```python
from build123d import *

# Parameters (mm, degrees)
F1_DEPTH = 15


with BuildPart() as f1:
    # F0 (on Top) → F1 (new body)
    with BuildSketch(Plane.XY):
        with BuildLine():
            Line((-28, 8), (-28, 0))
            Line((-28, 0), (22, 0))
            Line((22, 0), (22, 8))
            ThreePointArc((22, 8), (21.414214, 9.414214), (20, 10))
            Line((20, 10), (12, 10))
            ThreePointArc((12, 10), (10.585786, 10.585786), (10, 12))
            Line((10, 12), (10, 31))
            ThreePointArc((10, 31), (6.485281, 39.485281), (-2, 43))
            Line((-2, 43), (-3.051823, 43))
            Line((-3.051823, 43), (-6, 43))
            ThreePointArc((-6, 43), (-14.485281, 39.485281), (-18, 31))
            Line((-18, 31), (-18, 27))
            ThreePointArc((-18, 27), (-16.828427, 24.171573), (-14, 23))
            ThreePointArc((-14, 23), (-11.171573, 24.171573), (-10, 27))
            Line((-10, 27), (-10, 31))
            ThreePointArc((-10, 31), (-8.828427, 33.828427), (-6, 35))
            Line((-6, 35), (-2, 35))
            ThreePointArc((-2, 35), (0.828427, 33.828427), (2, 31))
            Line((2, 31), (2, 22))
            ThreePointArc((2, 22), (-1.514719, 13.514719), (-10, 10))
            Line((-10, 10), (-26, 10))
            ThreePointArc((-26, 10), (-27.414214, 9.414214), (-28, 8))
        make_face()
    extrude(amount=F1_DEPTH)


solid = f1.part
```
Source: CAD feature listing. Evaluate the final solid. Frame: model axes, mm. A direction names the side the tool comes from. Give positions to 0.01 mm unless a question says otherwise; leave off trailing zeros. Order: outer loops, then holes, each group sorted by start corner. A loop starts at its lowest first (then second) coordinate and runs counter-clockwise, first axis right, second up.
(1) Section query A-A (y = 28). Return the cut outline in (x, z), plus the area to 3 significant figures.
(2) Contact query for flat-ended pins moving along their axis: P1, Ø1, axis at y = 29, z = 1.5, coming from the -X side; P2, Ø4.5, axis at x = -18.5, z = 8.5, coming from the +Y side; P3, Ø4, axis at x = 2, z = 4, coming from the +Y side; P4, Ø10, axis at x = -16, y = 14, coming from the +Z side. Output: stop coordinate, or through.
(3) Access query for faces 1 (the face through (-18, 29, 7)), 2 (the face through (-10, 29, 7)), 3 (the face through (16, 10, 7)), 4 (the face through (-18, 10, 7)). Directions: +Z, -Z, +X, -X, +Y, -Y. A direction counts if a zero-diameter tool reaches every point of the face in a straight line with its end or side. Return the directions, or none.
(4) Section query D-D (x = -24.5). Return the cut outline in (y, z).
(5) Material intervals for line 1 along X through (y, z) = (29, 8.25); line 2 along Y through (x, z) = (12, 12.75); line 3 along Y through (x, z) = (-2, 7.5), sorted ascending.
(6) Section query B-B (x = -7). Return the cut outline in (y, z), plus the area to 3 significant figures.
(7) Pull-direction query (Y, two-part tool) for faces 5 (the face through (2, 17, 15)), 6 (the face through (-1.42, 13.61, 7.4)), 7 (the face through (-27.4, 9.43, 7.4)); classes: +Y half, -Y half, draft (parallel to the pull), parting line (faces both ways), or undercut.
(8) Section query C-C (z = 4.75). Return the cut outline in (x, y), plus the area to 3 significant figures.
Outcome:
1. outline: (-18, 0) - (-10, 0) - (-10, 15) - (-18, 15) - close; (2, 0) - (10, 0) - (10, 15) - (2, 15) - close
1. area: 240 mm2
2. P1: stops at x = -18
2. P2: stops at y = 37.24
2. P3: stops at y = 42.83
2. P4: stops at z = 15
3. face 1: +Z, -Z, -X, +Y
3. face 2: +Z, -Z
3. face 3: +Z, -Z, +X, +Y
3. face 4: +Z, -Z, -X
4. outline: (0, 0) - (10, 0) - (10, 15) - (0, 15) - close
5. line 1: x = -18 to -10, 2 to 10
5. line 2: y = 0 to 10
5. line 3: y = 0 to 13.06, 35 to 43
6. outline: (0, 0) - (10.38, 0) - (10.38, 15) - (0, 15) - close; (34.87, 0) - (42.96, 0) - (42.96, 15) - (34.87, 15) - close
6. area: 277 mm2
7. face 5: draft
7. face 6: undercut
7. face 7: +Y half
8. outline: (-28, 0) - (22, 0) - (22, 8) arc R2 ccw to (20, 10) - (12, 10) arc R2 cw to (10, 12) - (10, 31) arc R12 ccw to (-2, 43) - (-6, 43) arc R12 ccw to (-18, 31) - (-18, 27) arc R4 ccw to (-10, 27) - (-10, 31) arc R4 cw to (-6, 35) - (-2, 35) arc R4 cw to (2, 31) - (2, 22) arc R12 cw to (-10, 10) - (-26, 10) arc R2 ccw to (-28, 8) - close
8. area: 988 mm2
